Input: part model. Units: mm. Frame: model coordinates. Face numbers are marked on the shaded views. A direction names the side the tool comes from. Give positions to 0.01 mm unless a question says otherwise; leave off trailing zeros. Write each loop counter-clockwise with the first axis right and the second up, starting at its lowest first coordinate (ties: lowest second). Pieces come first, ordered by that corner, then holes. Notation, with made-up numbers: (67, 27) - (90, 27) arc R14 ccw to (90, 36) - close; hole circle Ø9 at (19.5, 20). An arc over 180 degrees is marked (long way). Answer as a JSON object with one key per item and string values. Group by question number.
from build123d import *

# Parameters (mm, degrees)
F1_DEPTH = 7.9375
F2_R     = 1.5512489022
F3_DEPTH = 3.175
F4_R     = 3.175
F5_DEPTH = 25.4
F6_R     = 3.96874


# Not quite as in the source:
# - a fillet or chamfer is up to 0.001 mm smaller than in the source, because OpenCascade refuses the exact size


with BuildPart() as f1:
    # F0 (on Top) → F1 (new body)
    with BuildSketch(Plane.XY):
        with BuildLine():
            Line((-9.9351188985, 0), (0, 0))
            ThreePointArc((0, 0), (6.3438186296, 3.1635706978), (12.2898811015, -0.6960349097))
            Line((12.2898811015, -0.6960349097), (15.4648811015, -0.6960349097))
            ThreePointArc((15.4648811015, -0.6960349097), (21.8148811015, 3.175), (28.1648811015, -0.6960349097))
            Line((28.1648811015, -0.6960349097), (31.3398811015, -0.6960349097))
            ThreePointArc((31.3398811015, -0.6960349097), (37.6898811015, 3.175), (44.0398811015, -0.6960349097))
            Line((44.0398811015, -0.6960349097), (47.2148811015, -0.6960349097))
            ThreePointArc((47.2148811015, -0.6960349097), (53.1609435734, 3.1635706978), (59.504762203, 0))
            Line((59.504762203, 0), (69.4398811015, 0))
            Line((69.4398811015, 0), (69.4398811015, 3.175))
            Line((69.4398811015, 3.175), (61.0109161202, 3.175))
            ThreePointArc((61.0109161202, 3.175), (53.1959495352, 6.3434025911), (45.6273811015, 2.6246326912))
            ThreePointArc((45.6273811015, 2.6246326912), (37.6898811015, 6.35), (29.7523811015, 2.6246326912))
            ThreePointArc((29.7523811015, 2.6246326912), (21.8148811015, 6.35), (13.8773811015, 2.6246326912))
            ThreePointArc((13.8773811015, 2.6246326912), (6.3088126678, 6.3434025911), (-1.5061539172, 3.175))
            Line((-1.5061539172, 3.175), (-9.9351188985, 3.175))
            Line((-9.9351188985, 3.175), (-9.9351188985, 0))
        make_face()
    extrude(amount=F1_DEPTH)

    # F2 (on face) → F3 (cut, through all)
    with BuildSketch(Plane(origin=(0, 3.175, 0), x_dir=(-1, 0, 0), z_dir=(0, 1, 0))):
        with Locations((5.9663688985, 3.96875)):
            Circle(F2_R)
        with Locations((-65.4711311015, 3.96875)):
            Circle(F2_R)
    extrude(amount=-F3_DEPTH, mode=Mode.SUBTRACT)

    # F4 (on face) → F5 (cut)
    with BuildSketch(Plane(origin=(0, 3.175, 0), x_dir=(-1, 0, 0), z_dir=(0, 1, 0))):
        with Locations((5.9663688985, 3.96875)):
            Circle(F4_R)
        with Locations((-65.4711311015, 3.96875)):
            Circle(F4_R)
    extrude(amount=F5_DEPTH, mode=Mode.SUBTRACT)

    # F6 (radius 3.96875 in the source; OpenCascade refuses exactly that, so slightly less here)
    f6_edges = [f1.edges().sort_by_distance(p)[0] for p in [
        (69.439881, 1.5875, 7.9375),
        (69.439881, 1.5875, 0),
        (-9.935119, 1.5875, 7.9375),
        (-9.935119, 1.5875, 0),
    ]]
    fillet(f6_edges, radius=F6_R)


solid = f1.part
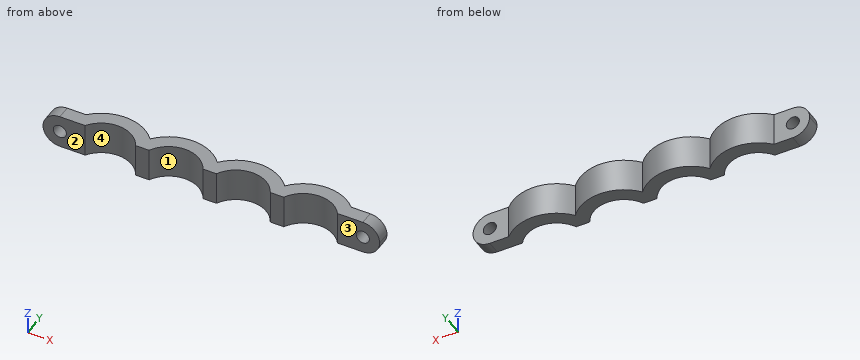
1) Reachability of the marked faces 3 and 4 from +Z, -Z, +X, -X, +Y, -Y: full face, straight path, thin tool, end or side. Return the list, or none.
2) Cut plane C-C on z = 0.75. Return the cut outline in (x, y) (1 decimal), and give its area (3 significant figures).
3) Mould query, pull axis X, two halves, no side actions, for the marked faces 1 and 2. Classes: +X half, -X half, draft (parallel to the pull), parting line (faces both ways), or undercut.
4) Cut plane D-D on x = -3. Return the cut outline in (y, z) (1 decimal), and give its area (3 significant figures).
5) Cut plane B-B on y = 5.5. Return the cut outline in (x, z), and give its area (3 significant figures).
6) Pin query (flat end, axial travel): P1, Ø4, axis at y = 4.5, z = 1.5, coming from the +X side; P2, Ø1.5, axis at x = 43.5, z = 5, coming from the +Y side; P3, Ø1.5, axis at x = 56, z = 5.5, coming from the +Y side. Return the tip coordinate at first contact, or that it passes through.
7) Cut plane A-A on y = 1.75. Count the separate pieces of the cut face and the enclosed holes in it, and give its area (3 significant figures).
8) Line query: line 1 along X through (y, z) = (3.25, 3.75); line 2 along Y through (x, z) = (53.5, 6.75); line 3 along X through (y, z) = (5, 0.75). Output: solid intervals per line, ascending. Write a range as from..to.
Filled in:
{
 "1": {"face 3": "+Z, -Z, +X, -Y", "face 4": "+Z, -Z, -Y"},
 "2": {"outline": "(-8.3, 0) - (0, 0) arc R7.1 cw to (12.3, -0.7) - (15.5, -0.7) arc R7.1 cw to (28.2, -0.7) - (31.3, -0.7) arc R7.1 cw to (44, -0.7) - (47.2, -0.7) arc R7.1 cw to (59.5, 0) - (67.8, 0) - (67.8, 3.2) - (61, 3.2) arc R10.3 ccw to (45.6, 2.6) arc R10.3 ccw to (29.8, 2.6) arc R10.3 ccw to (13.9, 2.6) arc R10.3 ccw to (-1.5, 3.2) - (-8.3, 3.2) - close", "area": "273 mm²"},
 "3": {"face 1": "undercut", "face 2": "draft"},
 "4": {"outline": "(0, 0) - (3.2, 0) - (3.2, 7.9) - (0, 7.9) - close", "area": "25.2 mm²"},
 "5": {"outline": "(1.84, 0) - (10.04, 0) - (10.04, 7.94) - (1.84, 7.94) - close; (17.71, 0) - (25.92, 0) - (25.92, 7.94) - (17.71, 7.94) - close; (33.59, 0) - (41.79, 0) - (41.79, 7.94) - (33.59, 7.94) - close; (49.46, 0) - (57.67, 0) - (57.67, 7.94) - (49.46, 7.94) - close", "area": "260 mm²"},
 "6": {"P1": "stops at x = 69.32", "P2": "stops at y = 5.02", "P3": "stops at y = 6.21"},
 "7": {"separate pieces": "5", "enclosed holes": "2", "area": "330 mm²"},
 "8": {"line 1": "x = -1.43..13.31, 14.44..29.19, 30.32..45.06, 46.19..60.94", "line 2": "y = 3.17..6.35", "line 3": "x = 0.84..11.04, 16.71..26.92, 32.59..42.79, 48.46..58.67"}
}
